The listing builds one solid part. Answer for the finished solid, in the listing's coordinates (mm). Face numbers are marked on the shaded views. Coordinates: 2 decimals unless noted, no trailing zeros. Write each loop counter-clockwise with the first axis right and the second up, starting at its lowest first coordinate (ties: lowest second). Pieces come first, ordered by that corner, then holes.
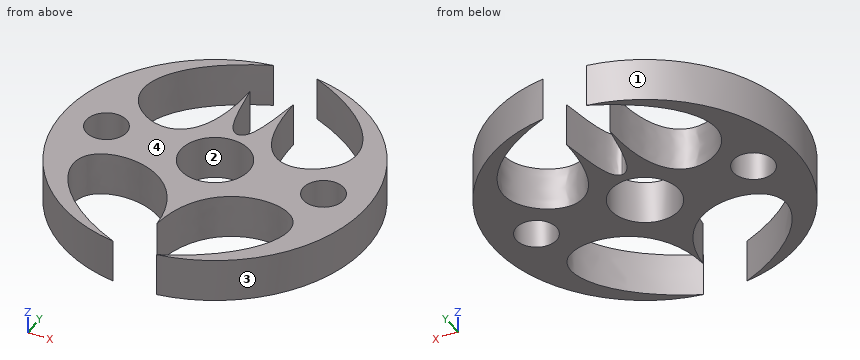
from build123d import *

# Parameters (mm, degrees)
F0_R     = 2.9614248249
F1_DEPTH = 6.35
F4_D     = 10


with BuildPart() as f1:
    # F0 (on Top) → F1 (new body)
    with BuildSketch(Plane.XY):
        with BuildLine():
            add(Edge.make_bspline(
                [(-3.175, 21.9970452561), (-13.4701055795, 17.6778641435), (-21.5584756618, 5.0746489519), (-3.175, 0), (-3.175, 15.5542598667)],
                knots=[0, 0, 0, 0, 0.5348418709, 1, 1, 1, 1], degree=3))
            ThreePointArc((-3.175, 21.9970452561), (-22.225, 0), (-3.175, -21.9970452561))
            add(Edge.make_bspline(
                [(-3.175, -21.9970452561), (-13.8975393501, -17.343846892), (-22.0709782387, -2.0584159269), (-0.8734419243, -4.604915157), (0, -15.875)],
                knots=[0, 0, 0, 0, 0.5133101899, 1, 1, 1, 1], degree=3))
            Line((0, -15.875), (0, 6.35))
            add(Edge.make_bspline(
                [(-3.175, 15.5542598667), (-2.5128191337, 11.9973989204), (-2.0055109635, 6.35), (0, 6.35)],
                knots=[0, 0, 0, 0, 9.7364790707, 9.7364790707, 9.7364790707, 9.7364790707], degree=3))
        make_face()
        with Locations((-15.875, 0)):
            Circle(F0_R, mode=Mode.SUBTRACT)
    extrude(amount=F1_DEPTH)

    # F2: F1 across face


with BuildPart() as f1_1:
    add(f1.part)
    add(f1.part.mirror(Plane(origin=(0, -4.7625, 3.175), x_dir=(0, 1, 0), z_dir=(1, 0, 0))))

    # F4 (through all)
    with Locations(Plane.XY.offset(6.35)):
        with Locations((0, 0)):
            Hole(F4_D / 2)


solid = f1_1.part
1. For a pull along X with two mould halves and no side action, classify the marked faces 1, 2, 3 and 4 as pulls with the +X half, pulls with the -X half, needs draft (parallel to the pull), parting line crosses it, or undercut.
Results found:
face 1: pulls with the -X half
face 2: undercut
face 3: pulls with the +X half
face 4: needs draft
2. Section A-A on y = 2 is taken. Give the vertices of the cut face in (x, z), then the cut area to 3 significant figures.
Results found:
outline: (-22.13, 0) - (-18.06, 0) - (-18.06, 6.35) - (-22.13, 6.35) - close; (-13.69, 0) - (-4.58, 0) - (-4.58, 6.35) - (-13.69, 6.35) - close; (4.58, 0) - (13.69, 0) - (13.69, 6.35) - (4.58, 6.35) - close; (18.06, 0) - (22.13, 0) - (22.13, 6.35) - (18.06, 6.35) - close
area: 167 mm2
3. Find the intervals of material crossed by L1, parallel to Y at x = 6.5, z = 1.5; L2, parallel to Y at x = -9, z = 5.25; L3, parallel to X at y = -8, z = 1.5, in increasing order.
Results found:
L1: y = -21.25 to -20.34, -5.7 to 4.34, 20.41 to 21.25
L2: y = -20.32 to -18.76, -5.04 to 3.39, 18.9 to 20.32
L3: x = -20.74 to -15.61, -3.15 to 3.15, 15.61 to 20.74
4. Flat-ended cylindrical pins translate along their axes: P1, Ø2, axis at y = -16, z = 2.5, coming from the -X side; P2, Ø1.5, axis at x = 5.5, z = 4, coming from the -Y side; P3, Ø1.5, axis at y = -8, z = 2, coming from the -X side; P4, Ø5, axis at x = 5.5, y = -13.5, coming from the +Z side. Find the tip coordinate at first contact, or state that the pin passes through.
Results found:
P1: stops at x = -16.4
P2: stops at y = -21.71
P3: stops at x = -21.01
P4: passes through
5. Section B-B on y = -11 is taken. State how many separate pieces and enclosed holes the cut face has, then the cut area to 3 significant figures.
Results found:
separate pieces: 3
enclosed holes: 0
area: 63.4 mm2
